Check sheet for the modelled part. Datum: model origin and axes. Units: mm. A direction names the side the tool comes from. Coordinates: 2 decimals unless noted, no trailing zeros. Loops run counter-clockwise (first coordinate to the right, second up) from the corner with the lowest first, then second, coordinate; pieces in that order, holes last.
from build123d import *

# Parameters (mm, degrees)
F0_R     = 381
F1_DEPTH = 254
F2_R     = 203.2
F3_DEPTH = 271.78
F4_T     = -9
F5_R     = 20
F6_R     = 8
F7_R     = 5
F8_DEPTH = 9


with BuildPart() as f1:
    # F0 (on Front) → F1 (new body)
    with BuildSketch(Plane.XZ):
        Circle(F0_R)
    extrude(amount=F1_DEPTH)

    # F2 (on face) → F3 (cut)
    with BuildSketch(Plane.XZ.offset(254)):
        Circle(F2_R)
    extrude(amount=-F3_DEPTH, mode=Mode.SUBTRACT)

    # F4
    f4_openings = [f1.faces().sort_by_distance(p)[0] for p in [
        (-203.2, -127, 0),
    ]]
    offset(amount=F4_T, openings=f4_openings)

    # F5
    f5_edges = [f1.edges().sort_by_distance(p)[0] for p in [
        (-381, -254, 0),
        (-381, 0, 0),
    ]]
    fillet(f5_edges, radius=F5_R)

    # F6
    f6_edges = [f1.edges().sort_by_distance(p)[0] for p in [
        (-203.2, -254, 0),
        (-203.2, 0, 0),
    ]]
    fillet(f6_edges, radius=F6_R)

    # F7 (on face) → F8 (cut, through all)
    with BuildSketch(Plane.XZ.offset(254)):
        with Locations((0, 231.2)):
            Circle(F7_R)
        with Locations((-71.444729, 219.884267)):
            Circle(F7_R)
        with Locations((-135.89595, 187.044729)):
            Circle(F7_R)
        with Locations((-187.044729, 135.89595)):
            Circle(F7_R)
        with Locations((-219.884267, 71.444729)):
            Circle(F7_R)
        with Locations((-231.2, 0)):
            Circle(F7_R)
        with Locations((-219.884267, -71.444729)):
            Circle(F7_R)
        with Locations((-187.044729, -135.89595)):
            Circle(F7_R)
        with Locations((-135.89595, -187.044729)):
            Circle(F7_R)
        with Locations((-71.444729, -219.884267)):
            Circle(F7_R)
        with Locations((0, -231.2)):
            Circle(F7_R)
        with Locations((71.444729, -219.884267)):
            Circle(F7_R)
        with Locations((135.89595, -187.044729)):
            Circle(F7_R)
        with Locations((187.044729, -135.89595)):
            Circle(F7_R)
        with Locations((219.884267, -71.444729)):
            Circle(F7_R)
        with Locations((231.2, 0)):
            Circle(F7_R)
        with Locations((219.884267, 71.444729)):
            Circle(F7_R)
        with Locations((187.044729, 135.89595)):
            Circle(F7_R)
        with Locations((135.89595, 187.044729)):
            Circle(F7_R)
        with Locations((71.444729, 219.884267)):
            Circle(F7_R)
    extrude(amount=-F8_DEPTH, mode=Mode.SUBTRACT)


solid = f1.part
(1) Section check A-A, the plane y = -120.5. Enter the section's corners in (x, z).
(2) Scan lines: line 1 along Z through (x, y) = (0, -250); line 2 along X through (y, z) = (-64, 1.5); line 3 along Y through (x, z) = (268, -112). Record each from-to range of solid material in increasing order.
(3) Gauge pin test, flat ends, axial feed: P1, Ø16, axis at x = 0, z = -231.2, coming from the -Y side; P2, Ø12, axis at x = -86.5, y = -151.5, coming from the -Z side; P3, Ø6, axis at x = -71.44, z = 219.88, coming from the -Y side; P4, Ø1, axis at y = -98, z = -250, coming from the +X side. Record the tip position at first contact, or that the pin passes through.
(4) Set-up check for faces 4 (the face through (155, 0, -155)), 5 (the face through (160, -9, -160)): record each of +Z, -Z, +X, -X, +Y, -Y from which the full face is reachable in a straight line by a thin tool's end or side.
(5) Draft check along Z on faces 1 (the face through (155, -254, -155)), 2 (the face through (-302.35, -125.5, -231.83)), 3 (the face through (354.82, -125.35, 111.74)). Enter one of: pulls with the +Z half, pulls with the -Z half, needs draft (parallel to the pull), parting line crosses it, or undercut.
Determined:
1. outline: circle Ø762 at (0, 0); hole circle Ø744 at (0, 0)
2. line 1: z = -373 to -236.2, -226.2 to -204.27, 204.27 to 226.2, 236.2 to 373
2. line 2: x = -381 to -372, 372 to 381
2. line 3: y = -254 to -245, -9 to 0
3. P1: stops at y = -254
3. P2: stops at z = -372.4
3. P3: stops at y = -9
3. P4: stops at x = 287.94
4. face 4: +Z, -Z, +X, -X, +Y
4. face 5: none
5. face 1: needs draft
5. face 2: parting line crosses it
5. face 3: undercut
